Build history of the part. All positions in model axes, mm. A direction names the side the tool comes from. Round coordinates to 2 decimals unless told otherwise and drop trailing zeros. Order: outer loops, then holes, each group sorted by start corner. A loop starts at its lowest first (then second) coordinate and runs counter-clockwise, first axis right, second up. Notation, with made-up numbers: (-11, 57) -> (23, 57) arc R27 ccw to (23, 81) -> close; hole circle Ø8 at (-21, 41). An arc over 180 degrees is marked (long way). Write item = value, one per line.
from build123d import *

# Parameters (mm, degrees)
SKETCH1_W           = 150
SKETCH1_H           = 40
BOSS_EXTRUDE1_DEPTH = 2
SKETCH2_W           = 150
SKETCH2_H           = 2
BOSS_EXTRUDE2_DEPTH = 40
CUT_EXTRUDE2_DEPTH  = 10
CUT_EXTRUDE4_DEPTH  = 10


with BuildPart() as part:
    # Sketch1 → Boss-Extrude1 (new body)
    with BuildSketch(Plane(origin=(0, 0, 0), x_dir=(1, 0, 0), z_dir=(0, 1, 0))):
        Rectangle(SKETCH1_W, SKETCH1_H)
    extrude(amount=BOSS_EXTRUDE1_DEPTH)

    # Sketch2 → Boss-Extrude2 (add)
    with BuildSketch(Plane(origin=(0, 2, 0), x_dir=(1, 0, 0), z_dir=(0, 1, 0))):
        with Locations((0, -19)):
            Rectangle(SKETCH2_W, SKETCH2_H)
    extrude(amount=BOSS_EXTRUDE2_DEPTH)

    # Sketch3 → Cut-Extrude2 (cut)
    with BuildSketch(Plane.XY.offset(20)):
        with BuildLine():
            Line((-36.788952994, 24.648821368), (-21.788952994, 24.648821368))
            ThreePointArc((-21.788952994, 24.648821368), (-18.13017777, 20.990046144), (-21.788952994, 17.33127092))
            Line((-21.788952994, 17.33127092), (-36.788952994, 17.33127092))
            ThreePointArc((-36.788952994, 17.33127092), (-40.447728218, 20.990046144), (-36.788952994, 24.648821368))
        make_face()
        with BuildLine():
            Line((-66.788952994, 24.648821368), (-51.788952994, 24.648821368))
            ThreePointArc((-51.788952994, 24.648821368), (-48.13017777, 20.990046144), (-51.788952994, 17.33127092))
            Line((-51.788952994, 17.33127092), (-66.788952994, 17.33127092))
            ThreePointArc((-66.788952994, 17.33127092), (-70.447728218, 20.990046144), (-66.788952994, 24.648821368))
        make_face()
        with BuildLine():
            Line((-6.788952994, 24.648821368), (8.211047006, 24.648821368))
            ThreePointArc((8.211047006, 24.648821368), (11.86982223, 20.990046144), (8.211047006, 17.33127092))
            Line((8.211047006, 17.33127092), (-6.788952994, 17.33127092))
            ThreePointArc((-6.788952994, 17.33127092), (-10.447728218, 20.990046144), (-6.788952994, 24.648821368))
        make_face()
        with BuildLine():
            Line((23.211047006, 24.648821368), (38.211047006, 24.648821368))
            ThreePointArc((38.211047006, 24.648821368), (41.86982223, 20.990046144), (38.211047006, 17.33127092))
            Line((38.211047006, 17.33127092), (23.211047006, 17.33127092))
            ThreePointArc((23.211047006, 17.33127092), (19.552271782, 20.990046144), (23.211047006, 24.648821368))
        make_face()
        with BuildLine():
            Line((53.211047006, 24.648821368), (68.211047006, 24.648821368))
            ThreePointArc((68.211047006, 24.648821368), (71.86982223, 20.990046144), (68.211047006, 17.33127092))
            Line((68.211047006, 17.33127092), (53.211047006, 17.33127092))
            ThreePointArc((53.211047006, 17.33127092), (49.552271782, 20.990046144), (53.211047006, 24.648821368))
        make_face()
    extrude(amount=-CUT_EXTRUDE2_DEPTH, mode=Mode.SUBTRACT)

    # Sketch4 → Cut-Extrude4 (cut)
    with BuildSketch(Plane.XZ):
        with BuildLine():
            Line((-35.090017562, 3.65), (-20.090017562, 3.65))
            ThreePointArc((-20.090017562, 3.65), (-16.440017562, 0), (-20.090017562, -3.65))
            Line((-20.090017562, -3.65), (-35.090017562, -3.65))
            ThreePointArc((-35.090017562, -3.65), (-38.740017562, 0), (-35.090017562, 3.65))
        make_face()
        with BuildLine():
            Line((-65.090017562, 3.65), (-50.090017562, 3.65))
            ThreePointArc((-50.090017562, 3.65), (-46.440017562, 0), (-50.090017562, -3.65))
            Line((-50.090017562, -3.65), (-65.090017562, -3.65))
            ThreePointArc((-65.090017562, -3.65), (-68.740017562, 0), (-65.090017562, 3.65))
        make_face()
        with BuildLine():
            Line((-5.090017562, 3.65), (9.909982438, 3.65))
            ThreePointArc((9.909982438, 3.65), (13.559982438, 0), (9.909982438, -3.65))
            Line((9.909982438, -3.65), (-5.090017562, -3.65))
            ThreePointArc((-5.090017562, -3.65), (-8.740017562, 0), (-5.090017562, 3.65))
        make_face()
        with BuildLine():
            Line((24.909982438, 3.65), (39.909982438, 3.65))
            ThreePointArc((39.909982438, 3.65), (43.559982438, 0), (39.909982438, -3.65))
            Line((39.909982438, -3.65), (24.909982438, -3.65))
            ThreePointArc((24.909982438, -3.65), (21.259982438, 0), (24.909982438, 3.65))
        make_face()
        with BuildLine():
            Line((54.909982438, 3.65), (69.909982438, 3.65))
            ThreePointArc((69.909982438, 3.65), (73.559982438, 0), (69.909982438, -3.65))
            Line((69.909982438, -3.65), (54.909982438, -3.65))
            ThreePointArc((54.909982438, -3.65), (51.259982438, 0), (54.909982438, 3.65))
        make_face()
    extrude(amount=-CUT_EXTRUDE4_DEPTH, mode=Mode.SUBTRACT)


solid = part.part
Q1. Cut at A-A, the plane z = 0. List the corners of the cut face in (x, y).
Check values:
outline = (-75, 0) -> (-68.74, 0) -> (-68.74, 2) -> (-75, 2) -> close; (-46.44, 0) -> (-38.74, 0) -> (-38.74, 2) -> (-46.44, 2) -> close; (-16.44, 0) -> (-8.74, 0) -> (-8.74, 2) -> (-16.44, 2) -> close; (13.56, 0) -> (21.26, 0) -> (21.26, 2) -> (13.56, 2) -> close; (43.56, 0) -> (51.26, 0) -> (51.26, 2) -> (43.56, 2) -> close; (73.56, 0) -> (75, 0) -> (75, 2) -> (73.56, 2) -> close
Q2. Probe probe 1 along Y at (x, z) = (35.5, -5); probe 2 along Z at (x, y) = (-7.5, 40). List the from-to ranges inside material, lowest first.
Check values:
probe_1 = 0 to 2
probe_2 = 18 to 20
Q3. Mould opens along Y. For faces 1 (the face through (-70.447, 20.91, 19.014)), 2 (the face through (-1, 2, -5)), 3 (the face through (-16.44, 0.99, 0.08)) say: released by +Y, released by -Y, zero draft, split by the parting line, or undercut.
Check values:
face_1 = undercut
face_2 = released by +Y
face_3 = zero draft
Q4. Flat gauge pins, fed straight in: pin 1 (4 mm diameter, centred on x = 56.5, y = 33, fed in from -Z); pin 2 (8 mm diameter, centred on x = -28.5, z = 12, fed in from +Y). Where does each tip first touch, or does it go through?
Check values:
pin_1 = 18
pin_2 = 2
Q5. Which spindle directions (+Z, -Z, +X, -X, +Y, -Y) get a long thin tool onto all of the face, cutting with end or side? Do faces 4 (the face through (-48.13, 21.07, 19.01)), 5 (the face through (-1, 17, 18)), 6 (the face through (21.26, 0.99, -0.08)). Say none if no direction does.
Check values:
face_4 = +Z, -Z
face_5 = -Z, +X, -X, +Y
face_6 = +Y, -Y
Q6. Cut at B-B, the plane x = 61.5. List the corners of the cut face in (y, z).
Check values:
outline = (0, -20) -> (2, -20) -> (2, -3.65) -> (0, -3.65) -> close; (0, 3.65) -> (2, 3.65) -> (2, 18) -> (17.33, 18) -> (17.33, 20) -> (0, 20) -> close; (24.65, 18) -> (42, 18) -> (42, 20) -> (24.65, 20) -> close
Q7. Cut at C-C, the plane z = -14.5. List the corners of the cut face in (x, y), and give its area (3 significant figures).
Check values:
outline = (-75, 0) -> (75, 0) -> (75, 2) -> (-75, 2) -> close
area = 300 mm²
